Work out the finished part from the listing and answer in its coordinate system (mm). Round coordinates to 2 decimals unless told otherwise and drop trailing zeros. Loops run counter-clockwise (first coordinate to the right, second up) from the corner with the lowest first, then second, coordinate; pieces in that order, holes last. Notation, with made-up numbers: (84, -11) - (124, -11) arc R19 ccw to (124, 12) - close; hole circle Ø4 at (14.5, -31). An arc over 180 degrees is marked (long way). Return JSON: item names as keys, results as strings.
from build123d import *

# Parameters (mm, degrees)
F2_SIZE = 0.49999


# Not quite as in the source:
# - a fillet or chamfer is up to 0.001 mm smaller than in the source, because OpenCascade refuses the exact size


with BuildPart() as f1:
    # F0 (on Front) → F1 (revolve)
    with BuildSketch(Plane.XZ):
        Polygon((-31.5, 0), (0, 0), (0, 4), (-26.5, 4), (-26.5, 5), (-31.5, 5), align=None)
    revolve(axis=Axis((0, 0, 2), (0, 0, -1)))

    # F2 (size 0.5 in the source; OpenCascade refuses exactly that, so slightly less here)
    f2_edges = [f1.edges().sort_by_distance(p)[0] for p in [
        (26.5, 0, 4),
        (26.5, 0, 5),
        (31.5, 0, 5),
        (31.5, 0, 0),
    ]]
    chamfer(f2_edges, length=F2_SIZE)


solid = f1.part
1) Determine the mould class of faces 1 (the cylindrical face through (4.101, 31.232, 2.472)), 2 (the flat face through (0, 0, 4)), 3 (the flat face through (2, 28, 5)) for opening direction Y: pulls with the +Y half, pulls with the -Y half, needs draft (parallel to the pull), parting line crosses it, or undercut.
Verdict:
{"face 1": "parting line crosses it", "face 2": "undercut", "face 3": "needs draft"}
2) Flat-ended cylindrical pins translate along their axes: pin 1 (1 mm diameter, centred on x = 3.5, z = 2.5, fed in from -Y); pin 2 (1.5 mm diameter, centred on x = -18, z = 3.5, fed in from +Y); pin 3 (15.5 mm diameter, centred on x = 10, y = 7, fed in from +Z). Find the tip coordinate at first contact, or state that the pin passes through.
Verdict:
{"pin 1": "stops at y = -31.36", "pin 2": "stops at y = 26.36", "pin 3": "stops at z = 4"}
3) Find the intervals of material crossed by L1, parallel to Z at x = 13.5, y = 15.5; L2, parallel to Y at x = 0, z = 4.5; L3, parallel to Y at x = -5.5, z = 3.9, in increasing order.
Verdict:
{"L1": "z = 0 to 4", "L2": "y = -31.5 to -26.5, 26.5 to 31.5", "L3": "y = -31.02 to 31.02"}
4) Section C-C (z = 1.9) is taken. Give the vertices of the cut face in (x, y), and give its area (3 significant figures).
Verdict:
{"outline": "circle Ø63 at (0, 0)", "area": "3,120 mm2"}
